```python
from build123d import *

# Parameters (mm, degrees)
BOSS_EXTRUDE1_DEPTH = 3
SKETCH2_W           = 3.6
SKETCH2_H           = 12
SKETCH2_H_2         = 6.5
CUT_EXTRUDE1_DEPTH  = 10


with BuildPart() as part:
    # Sketch1 → Boss-Extrude1 (new body)
    with BuildSketch(Plane(origin=(0, 0, 0), x_dir=(1, 0, 0), z_dir=(0, 1, 0))):
        Polygon((0, 0), (0, 15.5), (3, 15.5), (3, 25.5), (0, 25.5), (0, 35.5), (3, 35.5), (3, 45.5), (0, 45.5), (0, 55.5), (3, 55.5), (3, 65.5), (0, 65.5), (0, 75.5), (3, 75.5), (3, 85.5), (0, 85.5), (0, 95.5), (3, 95.5), (3, 105.5), (0, 105.5), (0, 115.5), (3, 115.5), (3, 125.5), (0, 125.5), (0, 135.5), (3, 135.5), (3, 145.5), (0, 145.5), (0, 155.5), (3, 155.5), (3, 165.5), (0, 165.5), (0, 181), (4.93, 181), (4.93, 178), (14.93, 178), (14.93, 181), (24.93, 181), (24.93, 178), (34.93, 178), (34.93, 181), (44.93, 181), (44.93, 178), (54.93, 178), (54.93, 181), (64.93, 181), (64.93, 178), (74.93, 178), (74.93, 181), (84.93, 181), (84.93, 178), (94.93, 178), (94.93, 181), (104.93, 181), (104.93, 178), (114.93, 178), (114.93, 181), (124.93, 181), (124.93, 178), (134.93, 178), (134.93, 181), (144.93, 181), (144.93, 0), (134.93, 0), (134.93, 3), (124.93, 3), (124.93, 0), (114.93, 0), (114.93, 3), (104.93, 3), (104.93, 0), (94.93, 0), (94.93, 3), (84.93, 3), (84.93, 0), (74.93, 0), (74.93, 3), (64.93, 3), (64.93, 0), (54.93, 0), (54.93, 3), (44.93, 3), (44.93, 0), (34.93, 0), (34.93, 3), (24.93, 3), (24.93, 0), (14.93, 0), (14.93, 3), (4.93, 3), (4.93, 0), align=None)
    extrude(amount=BOSS_EXTRUDE1_DEPTH)

    # Sketch2 → Cut-Extrude1 (cut)
    with BuildSketch(Plane.XZ):
        with Locations((63.13, -36)):
            Rectangle(SKETCH2_W, SKETCH2_H)
        with Locations((63.13, -12)):
            Rectangle(SKETCH2_W, SKETCH2_H)
        with Locations((63.13, -169)):
            Rectangle(SKETCH2_W, SKETCH2_H)
        with Locations((63.13, -145)):
            Rectangle(SKETCH2_W, SKETCH2_H)
        with Locations((63.13, -121)):
            Rectangle(SKETCH2_W, SKETCH2_H)
        with Locations((63.13, -99.75)):
            Rectangle(SKETCH2_W, SKETCH2_H_2)
        with Locations((63.13, -81.25)):
            Rectangle(SKETCH2_W, SKETCH2_H_2)
        with Locations((63.13, -60)):
            Rectangle(SKETCH2_W, SKETCH2_H)
    extrude(amount=-CUT_EXTRUDE1_DEPTH, mode=Mode.SUBTRACT)


solid = part.part
```
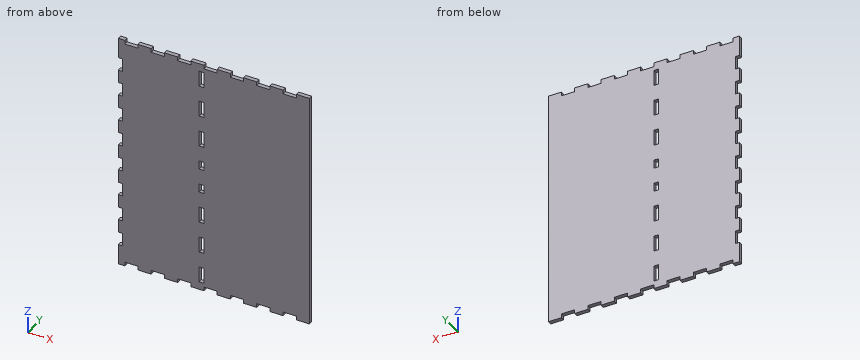
Build history of the part. All positions in model axes, mm. Coordinates: 2 decimals unless noted, no trailing zeros. Order: outer loops, then holes, each group sorted by start corner. A loop starts at its lowest first (then second) coordinate and runs counter-clockwise, first axis right, second up. Notation, with made-up numbers: (-37.75, -15) -> (-31.75, -15) arc R28 cw to (-31.75, 13) -> close; hole circle Ø1 at (29, -16.5). An arc over 180 degrees is marked (long way). Answer in a Markdown table with one row per item. Add a question column.
Q1. Band-saw the part on B-B, the plane x = 108. List the corners of the cut face in (y, z).
Q2. Band-saw the part on A-A, the plane z = -63. List the corners of the cut face in (x, y), then the cut area to 3 significant figures.
Q3. Drop flat-ended pins along their axis: pin 1 (8 mm diameter, centred on x = 45, z = -58.5, fed in from -Y); pin 2 (0.9 mm diameter, centred on y = 2, z = -80, fed in from -X); pin 3 (0.9 mm diameter, centred on x = 128.5, y = 1.5, fed in from -Z). Give the stop position or say it passes through.
Q4. Band-saw the part on C-C, the plane y = 1.55. Give the number of separate pieces and of enclosed holes in the cut face, then the cut area to 3 significant figures.
Q5. Wall check: line 1 along X through (y, z) = (1, -147); line 2 along X through (y, z) = (0.75, -121.5); line 3 along Z through (x, y) = (130, 0.75). Give the ranges that are in metal, low to high. Write a range as [from, to].
Answers follow:
| question | item | result |
|---|---|---|
| 1 | outline | (0, -178) -> (3, -178) -> (3, -3) -> (0, -3) -> close |
| 2 | outline | (3, 0) -> (61.33, 0) -> (61.33, 3) -> (3, 3) -> close; (64.93, 0) -> (144.93, 0) -> (144.93, 3) -> (64.93, 3) -> close |
| 2 | area | 415 mm^2 |
| 3 | pin 1 | y = 0 |
| 3 | pin 2 | x = 3 |
| 3 | pin 3 | z = -178 |
| 4 | separate pieces | 1 |
| 4 | enclosed holes | 8 |
| 4 | area | 25,300 mm^2 |
| 5 | line 1 | [0, 61.33], [64.93, 144.93] |
| 5 | line 2 | [3, 61.33], [64.93, 144.93] |
| 5 | line 3 | [-178, -3] |
